Build history of the part. All positions in model axes, mm. Face numbers are marked on the shaded views. A direction names the side the tool comes from. Round coordinates to 2 decimals unless told otherwise and drop trailing zeros. Write each loop counter-clockwise with the first axis right and the second up, starting at its lowest first coordinate (ties: lowest second). Pieces come first, ordered by that corner, then holes.
1) Saw through at B-B (y = -1.95). Write the cut outline in (x, z).
2) Saw through at A-A (z = 7). Write the cut outline in (x, y).
3) Pull direction X, two halves, no side cores. Call the marked faces 1, 2 and 3: +X half, -X half, draft (parallel to the pull), parting line (faces both ways), or undercut.
4) Wall check: probe 1 along Y at (x, z) = (-28.5, -4.5); probe 2 along X at (y, z) = (-0.35, 1); probe 3 along Z at (x, y) = (-16, -0.5). Give the ranges that are in metal, low to high.
5) Which spindle directions (+Z, -Z, +X, -X, +Y, -Y) get a long thin tool onto all of the face, cutting with end or side? Do the marked faces 4, 5 and 6. Say none if no direction does.
6) Saw through at D-D (x = -19). Write the cut outline in (y, z), plus the area to 3 significant figures.
7) Saw through at C-C (x = 21.5). Write the cut outline in (y, z), plus the area to 3 significant figures.
8) Flat gauge pins, fed straight in: pin 1 (3.5 mm diameter, centred on x = 21.72, z = -4.32, fed in from -Y); pin 2 (6 mm diameter, centred on x = -5, z = 14, fed in from +Y); pin 3 (1.2 mm diameter, centred on y = -1, z = 2.5, fed in from -X); pin 4 (10 mm diameter, centred on x = 0, z = -0.5, fed in from -Y). Where does each tip first touch, or does it go through?
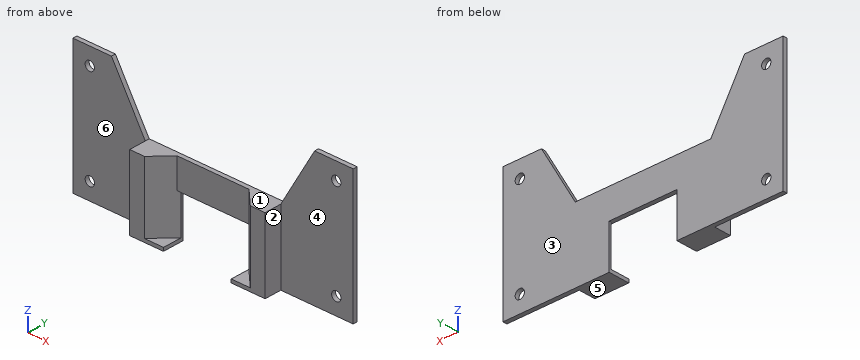
from build123d import *

# Parameters (mm, degrees)
SKETCH1_W             = 17.11
SKETCH1_H             = 31.14
SKETCH1_R             = 1.1
BOSS_EXTRUDE1_DEPTH   = 1
BOSS_EXTRUDE1_2_DEPTH = 1
SKETCH1_W_2           = 16
SKETCH1_H_2           = 7
BOSS_EXTRUDE1_3_DEPTH = 1
BOSS_EXTRUDE2_START   = 1
SKETCH1_3_W           = 8
SKETCH1_3_H           = 16.48
BOSS_EXTRUDE2_DEPTH   = 5
CHAMFER1_SIZE         = 4.5
CHAMFER2_SIZE         = 4.5
BOSS_EXTRUDE3_START   = 1
SKETCH1_4_W           = 8
SKETCH1_4_H           = 0.8
BOSS_EXTRUDE3_DEPTH   = 5
CHAMFER3_SIZE         = 8
CHAMFER3_SIZE2        = 13.856406461
CHAMFER4_SIZE         = 8
CHAMFER4_SIZE2        = 13.856406461


with BuildPart() as part:
    # Sketch1 → Boss-Extrude1 (new body)
    with BuildSketch(Plane(origin=(0, 0, 0), x_dir=(1, 0, 0), z_dir=(0, 1, 0))):
        with Locations((-31.94497183, -7.245370105)):
            Rectangle(SKETCH1_W, SKETCH1_H)
        with Locations((-36.49997183, -18.815370105)):
            Circle(SKETCH1_R, mode=Mode.SUBTRACT)
        with Locations((-36.49997183, 4.324629895)):
            Circle(SKETCH1_R, mode=Mode.SUBTRACT)
    extrude(amount=BOSS_EXTRUDE1_DEPTH)



with BuildPart() as body_2:
    # Sketch1 → Boss-Extrude1 2 (new body)
    with BuildSketch(Plane(origin=(0, 0, 0), x_dir=(1, 0, 0), z_dir=(0, 1, 0))):
        with Locations((17.16502817, -7.245370105)):
            Rectangle(SKETCH1_W, SKETCH1_H)
        with Locations((21.72002817, 4.324629895)):
            Circle(SKETCH1_R, mode=Mode.SUBTRACT)
        with Locations((21.72002817, -18.815370105)):
            Circle(SKETCH1_R, mode=Mode.SUBTRACT)
    extrude(amount=BOSS_EXTRUDE1_2_DEPTH)


with BuildPart() as body_3:
    # Sketch1 → Boss-Extrude1 3 (new body)
    with BuildSketch(Plane(origin=(0, 0, 0), x_dir=(1, 0, 0), z_dir=(0, 1, 0))):
        with Locations((-7.38997183, -5.455370105)):
            Rectangle(SKETCH1_W_2, SKETCH1_H_2)
    extrude(amount=BOSS_EXTRUDE1_3_DEPTH)


with BuildPart() as part_1:
    add(part.part)

    add(body_2.part)  # Boss-Extrude2 merges body 2

    add(body_3.part)  # Boss-Extrude2 merges body 3
    # Sketch1<3> → Boss-Extrude2 (add)
    with BuildSketch(Plane(origin=(0, 0, 0), x_dir=(1, 0, 0), z_dir=(0, 1, 0)).offset(BOSS_EXTRUDE2_START)):
        with Locations((-19.38997183, -0.715370105)):
            Rectangle(SKETCH1_3_W, SKETCH1_3_H)
        with Locations((4.61002817, -0.715370105)):
            Rectangle(SKETCH1_3_W, SKETCH1_3_H)
    extrude(amount=-BOSS_EXTRUDE2_DEPTH)

    # Chamfer1
    chamfer1_edges = [part_1.edges().sort_by_distance(p)[0] for p in [
        (0.61002817, -4, 0.715370105),
    ]]
    chamfer(chamfer1_edges, length=CHAMFER1_SIZE)

    # Chamfer2
    chamfer2_edges = [part_1.edges().sort_by_distance(p)[0] for p in [
        (-15.38997183, -4, 0.715370105),
    ]]
    chamfer(chamfer2_edges, length=CHAMFER2_SIZE)

    # Sketch1<4> → Boss-Extrude3 (add)
    with BuildSketch(Plane(origin=(0, 0, 0), x_dir=(1, 0, 0), z_dir=(0, 1, 0)).offset(BOSS_EXTRUDE3_START)):
        with Locations((-19.38997183, 7.924629895)):
            Rectangle(SKETCH1_4_W, SKETCH1_4_H)
        with Locations((4.61002817, 7.924629895)):
            Rectangle(SKETCH1_4_W, SKETCH1_4_H)
    extrude(amount=-BOSS_EXTRUDE3_DEPTH)

    # Chamfer3
    chamfer3_edges = [part_1.edges().sort_by_distance(p)[0] for p in [
        (-23.38997183, 0.5, 22.815370105),
    ]]
    chamfer3_side = [part_1.faces().sort_by_distance(p)[0] for p in [
        (-31.94497183, 0.5, 22.815370105),
    ]]
    chamfer(chamfer3_edges, length=CHAMFER3_SIZE, length2=CHAMFER3_SIZE2, reference=chamfer3_side[0])

    # Chamfer4
    chamfer4_edges = [part_1.edges().sort_by_distance(p)[0] for p in [
        (8.61002817, 0.5, 22.815370105),
    ]]
    chamfer4_side = [part_1.faces().sort_by_distance(p)[0] for p in [
        (17.16502817, 0.5, 22.815370105),
    ]]
    chamfer(chamfer4_edges, length=CHAMFER4_SIZE, length2=CHAMFER4_SIZE2, reference=chamfer4_side[0])


solid = part_1.part
Evaluation:
1. outline: (-23.39, -8.32) - (-15.39, -8.32) - (-15.39, -7.52) - (-17.84, -7.52) - (-17.84, 8.96) - (-23.39, 8.96) - close; (0.61, -8.32) - (8.61, -8.32) - (8.61, 8.96) - (3.06, 8.96) - (3.06, -7.52) - (0.61, -7.52) - close
2. outline: (-40.5, 0) - (-23.39, 0) - (-23.39, -4) - (-19.89, -4) - (-15.89, 0) - (1.11, 0) - (5.11, -4) - (8.61, -4) - (8.61, 0) - (25.72, 0) - (25.72, 1) - (-40.5, 1) - close
3. face 1: undercut
3. face 2: +X half
3. face 3: draft
4. probe 1: y = 0 to 1
4. probe 2: x = -23.39 to -16.24, 1.46 to 8.61
4. probe 3: z = -8.32 to -7.52
5. face 4: +Z, -Z, +X, -Y
5. face 5: -Z, +X, -X, +Y, -Y
5. face 6: +Z, -Z, -X, -Y
6. outline: (-4, -8.32) - (1, -8.32) - (1, 8.96) - (-3.11, 8.96) - (-3.11, -7.52) - (-4, -7.52) - close
6. area: 71.7 mm2
7. outline: (0, -8.32) - (1, -8.32) - (1, -5.4) - (0, -5.4) - close; (0, -3.25) - (1, -3.25) - (1, 17.74) - (0, 17.74) - close; (0, 19.89) - (1, 19.89) - (1, 22.82) - (0, 22.82) - close
7. area: 26.8 mm2
8. pin 1: stops at y = 0
8. pin 2: passes through
8. pin 3: stops at x = -23.39
8. pin 4: stops at y = -3.89
